Can you work these out from the model? Positions are in its coordinate system, mm. A direction names the side the tool comes from. Give positions to 0.01 mm unless a question says otherwise; leave off trailing zeros. Loops run counter-clockwise (first coordinate to the right, second up) from the corner with the lowest first, then second, coordinate; pieces in that order, holes last. Notation, with made-up numbers: (83, 43.25) - (110, 43.25) arc R8 cw to (110, 47.25) - close; hole circle Ø3 at (19.5, 51.5). An arc over 180 degrees is marked (long way). Answer as a JSON object with one key per item and string values. Group by question number.
Item 1: Please list where these lines run through material, in increasing order: L1, parallel to Y at x = 1.8, z = -24.5; L2, parallel to X at y = 3.35, z = -35; L3, parallel to Z at x = 1.2, y = 11.9.
Item 2: Suppose I cut it at D-D on x = 2.5. Write out the boundary of the cut face in (y, z), and give its area (3 significant figures).
Item 3: Will these pins go through, and if not, where does the flat tip stop? pin 1 (5 mm diameter, centred on x = 8.5, z = -7.5, fed in from +Y); pin 2 (6 mm diameter, centred on x = 12, y = 18.5, fed in from +Z); pin 3 (4 mm diameter, centred on y = 11.9, z = -24.5, fed in from +X).
Item 4: Suppose I cut it at A-A on z = -24.5. Write out the boundary of the cut face in (x, y), and give its area (3 significant figures).
Item 5: Which directions (+Z, -Z, +X, -X, +Y, -Y) give clear straight access to the entire face, cutting with the end or side of a thin tool? Please do faces 1 (the flat face through (6, 14, -10.5)), 2 (the flat face through (12, 5, -27)), 3 (the flat face through (2, 19, -29.5)), 4 (the cylindrical face through (18, 3, -39)).
Item 6: Thinking about a two-plate mould opening in Y: for faces 5 (the cylindrical face through (1.73, 28.2, -25.81)), 6 (the cylindrical face through (13.5, 2.5, -5.8)), 7 (the flat face through (10, 5, -5)), 8 (the cylindrical face through (1.73, 12.9, -23.19)), which applies, pulls with the +Y half, pulls with the -Y half, needs draft (parallel to the pull), parting line crosses it, or undercut?
Item 7: Suppose I cut it at C-C on y = 11.9. Write out the boundary of the cut face in (x, z).
Item 8: Suppose I cut it at B-B on x = 13. Write out the boundary of the cut face in (y, z).
from build123d import *

# Parameters (mm, degrees)
SKETCH_1_W          = 20
SKETCH_1_H          = 40
EXTRUDE_1_DEPTH     = 5
SKETCH_2_W          = 19
SKETCH_2_H          = 26.7
EXTRUDE_2_DEPTH     = 3.5
SKETCH_3_R          = 1.65
CUT_EXTRUDE_1_DEPTH = 55.816876963
SKETCH_4_R          = 1.7
CUT_EXTRUDE_2_DEPTH = 53.085410625
FILLET_1_R          = 5
FILLET_2_R          = 3
RIB_1_REACH         = 49.698
SKETCH_5_WALL_W     = 126.274874616
SKETCH_5_WALL_H     = 4
FILLET_3_R          = 5


with BuildPart() as part:
    # 草图1 → 凸台-拉伸1 (new body)
    with BuildSketch(Plane(origin=(0, 0, 0), x_dir=(1, 0, 0), z_dir=(0, 1, 0))):
        with Locations((10, 20)):
            Rectangle(SKETCH_1_W, SKETCH_1_H)
    extrude(amount=EXTRUDE_1_DEPTH)

    # 草图2 → 凸台-拉伸2 (add)
    with BuildSketch(Plane.ZY):
        with Locations((-20, 18.35)):
            Rectangle(SKETCH_2_W, SKETCH_2_H)
    extrude(amount=-EXTRUDE_2_DEPTH)

    # 草图3 → 切除-拉伸1 (cut, through all)
    with BuildSketch(Plane.ZY):
        with Locations((-24.5, 29.2)):
            Circle(SKETCH_3_R)
        with Locations(Location((-24.5, 11.9, 0), (0, 0, 180))):
            Circle(SKETCH_3_R)
    extrude(amount=-CUT_EXTRUDE_1_DEPTH, mode=Mode.SUBTRACT)

    # 草图4 → 切除-拉伸2 (cut, through all)
    with BuildSketch(Plane(origin=(0, 5, 0), x_dir=(1, 0, 0), z_dir=(0, 1, 0))):
        with Locations(Location((12, 35, 0), (0, 0, 270))):
            Circle(SKETCH_4_R)
        with Locations(Location((12, 5, 0), (0, 0, 90))):
            Circle(SKETCH_4_R)
    extrude(amount=-CUT_EXTRUDE_2_DEPTH, mode=Mode.SUBTRACT)

    # 圆角1
    fillet_1_edges = [part.edges().sort_by_distance(p)[0] for p in [
        (0, 2.5, -40),
        (20, 2.5, -40),
        (20, 2.5, 0),
        (0, 2.5, 0),
    ]]
    fillet(fillet_1_edges, radius=FILLET_1_R)

    # 圆角2
    fillet_2_edges = [part.edges().sort_by_distance(p)[0] for p in [
        (1.75, 31.7, -29.5),
        (1.75, 31.7, -10.5),
    ]]
    fillet(fillet_2_edges, radius=FILLET_2_R)

    # 草图5 wall → 筋1 (add, up to next)
    with BuildSketch(Plane(origin=(11.75, 16.85, -10.5), x_dir=(0.571368826083, -0.820693404738, 0), z_dir=(0.820693404738, 0.571368826083, 0)), mode=Mode.PRIVATE) as rib_1_sk1:
        with Locations((0, 2)):
            Rectangle(SKETCH_5_WALL_W, SKETCH_5_WALL_H)
    rib_1_tool1 = extrude(rib_1_sk1.sketch, amount=-RIB_1_REACH, mode=Mode.PRIVATE) - part.part
    add(rib_1_tool1.solids().sort_by_distance((11.75, 16.85, -10.5))[0])

    # 圆角3
    fillet_3_edges = [part.edges().sort_by_distance(p)[0] for p in [
        (1.75, 5, -29.5),
        (3.5, 5, -22),
        (3.5, 28.7, -12.5),
    ]]
    fillet(fillet_3_edges, radius=FILLET_3_R)


solid = part.part
Worked out:
{
 "1": {"L1": "y = 0 to 10.25, 13.55 to 27.55, 30.85 to 31.7", "L2": "x = 0 to 10.3, 13.7 to 20", "L3": "z = -29.5 to -26.15, -22.85 to -10.5"},
 "2": {"outline": "(0, -39.33) - (5, -39.33) - (5, -34.5) arc R5 cw to (10, -29.5) - (28.7, -29.5) arc R3 ccw to (31.7, -26.5) - (31.7, -13.5) arc R3 ccw to (28.7, -10.5) - (5, -10.5) - (5, -0.67) - (0, -0.67) - close; hole circle Ø3.3 at (11.9, -24.5); hole circle Ø3.3 at (29.2, -24.5)", "area": "685 mm2"},
 "3": {"pin 1": "stops at y = 5", "pin 2": "stops at z = -10.5", "pin 3": "stops at x = 3.5"},
 "4": {"outline": "(0, 0) - (20, 0) - (20, 5) - (8.5, 5) arc R5 cw to (3.5, 10) - (3.5, 10.25) - (0, 10.25) - close; (0, 13.55) - (3.5, 13.55) - (3.5, 27.55) - (0, 27.55) - close; (0, 30.85) - (3.5, 30.85) - (3.5, 31.7) - (0, 31.7) - close", "area": "176 mm2"},
 "5": {"face 1": "+Z, +X, -X, +Y", "face 2": "-Z, +X, +Y", "face 3": "-Z, +X, -X, +Y", "face 4": "-Z, +X, +Y, -Y"},
 "6": {"face 5": "undercut", "face 6": "needs draft", "face 7": "pulls with the +Y half", "face 8": "undercut"},
 "7": {"outline": "(0, -29.5) - (3.5, -29.5) - (3.5, -26.15) - (0, -26.15) - close; (0, -22.85) - (3.5, -22.85) - (3.5, -14.5) - (15.2, -14.5) - (15.2, -10.5) - (0, -10.5) - close"},
 "8": {"outline": "(0, -40) - (5, -40) - (5, -36.37) - (0, -36.37) - close; (0, -33.63) - (5, -33.63) - (5, -14.5) - (15.05, -14.5) - (15.05, -10.5) - (5, -10.5) - (5, -6.37) - (0, -6.37) - close; (0, -3.63) - (5, -3.63) - (5, 0) - (0, 0) - close"}
}
